For this review, take the finished solid that the model builds, in its own axes (mm). A direction names the side the tool comes from. Give positions to 0.01 mm unless a question says otherwise; leave off trailing zeros. Order: outer loops, then holes, each group sorted by start corner. A loop starts at its lowest first (then second) coordinate and runs counter-clockwise, first axis right, second up. Notation, with made-up numbers: (82, 7.5) -> (103, 7.5) arc R26 ccw to (103, 21.5) -> close; hole circle Ø6 at (-17, 39.25). An arc over 180 degrees is marked (long way). Return JSON: item names as keys, results as strings. Group by question number.
1) Add section A-A (z = 0). State how many separate pieces and enclosed holes the cut face has, then the cut area to 3 significant figures.
2) To check wall thickness, follow line 1 along X through (y, z) = (-8.15, 0) (3 decimals); line 2 along Y through (x, z) = (0, 2.35) (1 decimal); line 3 along X through (y, z) = (-8.5, 1.3). State the ranges of each line that lie inside material, in increasing order.
3) Add section B-B (y = -5.75). Give the boundary of the cut face in (x, z) (1 decimal), then the cut area to 3 significant figures.
4) Insertion check: P1, Ø3, axis at y = 4.5, z = 0, coming from the -X side; P2, Ø2, axis at y = -2, z = 0, coming from the +X side (3 decimals); P3, Ø3, axis at x = -5, z = 0.5, coming from the +Y side; P4, Ø1.9, axis at x = 14.29, z = 0, coming from the -Y side. Each pin has a flat end and moves straight along its axis. Give the tip position at first contact, or say it passes through.
5) For faces 1 (the face through (9.525, -2, 0)), 2 (the face through (-9.525, -2, 0)), 3 (the face through (-9.16, -1.72, 2.16)), 4 (the face through (-17.63, -7.11, -1.896)), 5 (the face through (9.16, -1.77, -2.16)), list the 3-axis set-ups (+Z, -Z, +X, -X, +Y, -Y) from which the entire face can be reached by the end or side of a thin tool; tool diameter is ignored.
from build123d import *

# Parameters (mm, degrees)
EXTRUDE1_DEPTH      = 2.54
EXTRUDE1_DEPTH_BACK = 2.54
SKETCH3_R           = 4.9784
SKETCH4_R           = 1.5875
CUT_EXTRUDE1_DEPTH  = 24.321126052
FILLET1_R           = 1.27
FILLET2_R           = 1.27
CHAMFER1_SIZE       = 0.127
FILLET3_R           = 0.254
CHAMFER2_SIZE       = 0.127


with BuildPart() as part:
    # Sketch3 → Extrude1 (new, two sides: drawn at the far end of the back side and taken through both)
    with BuildSketch(Plane.XY.offset(-EXTRUDE1_DEPTH_BACK)):
        with BuildLine():
            Line((9.525, 0), (9.525, -4.7625))
            Line((9.525, -4.7625), (18.25625, -4.7625))
            Line((18.25625, -4.7625), (18.25625, -9.525))
            Line((18.25625, -9.525), (-18.25625, -9.525))
            Line((-18.25625, -9.525), (-18.25625, -4.7625))
            Line((-18.25625, -4.7625), (-9.525, -4.7625))
            Line((-9.525, -4.7625), (-9.525, 0))
            ThreePointArc((-9.525, 0), (0, 9.525), (9.525, 0))
        make_face()
        Circle(SKETCH3_R, mode=Mode.SUBTRACT)
    extrude(amount=EXTRUDE1_DEPTH + EXTRUDE1_DEPTH_BACK)

    # Sketch4 → Cut-Extrude1 (cut, through all)
    with BuildSketch(Plane(origin=(0, -4.7625, 0), x_dir=(1, 0, 0), z_dir=(0, 1, 0))):
        with Locations(Location((-14.2875, 0, 0), (0, 0, 270))):
            Circle(SKETCH4_R)
        with Locations(Location((14.2875, 0, 0), (0, 0, 270))):
            Circle(SKETCH4_R)
        Polygon((-18.25625, 2.54), (-18.25625, 1.27), (-16.98625, 2.54), align=None)
        Polygon((16.98625, 2.54), (18.25625, 2.54), (18.25625, 1.27), align=None)
        Polygon((18.25625, -2.54), (18.25625, -1.27), (16.98625, -2.54), align=None)
        Polygon((-16.98625, -2.54), (-18.25625, -2.54), (-18.25625, -1.27), align=None)
    extrude(amount=-CUT_EXTRUDE1_DEPTH, mode=Mode.SUBTRACT)

    # Fillet1
    fillet1_edges = [part.edges().sort_by_distance(p)[0] for p in [
        (0, 9.525, -2.54),
        (9.525, -2.38125, -2.54),
        (9.525, -2.38125, 2.54),
        (-9.525, -2.38125, -2.54),
        (0, 9.525, 2.54),
        (-9.525, -2.38125, 2.54),
    ]]
    fillet(fillet1_edges, radius=FILLET1_R)

    # Fillet2
    # the kernel refuses this fillet: 1.27 mm, written as the material it adds along each edge
    with BuildSketch(Plane(origin=(-9.525, -4.7625, -1.27), x_dir=(0, 1, 0), z_dir=(0, 0, 1)), Plane(origin=(9.525, -4.7625, 1.27), x_dir=(0, 1, 0), z_dir=(0, 0, -1))) as fillet2_piece_1:
        with BuildLine():
            CenterArc((FILLET2_R, FILLET2_R), FILLET2_R, 180, 90)
            Line((0, FILLET2_R), (0, 0))
            Line((0, 0), (FILLET2_R, 0))
        make_face()
    extrude(amount=2.54)
    with BuildSketch(Plane(origin=(8.255, -4.7625, -1.27), x_dir=(-0.5976672776328268, 0, 0.8017442392976488), z_dir=(0.8017442392976488, 0, 0.5976672776328268))) as fillet2_piece_2_section:
        with BuildLine():
            CenterArc((1.27 + FILLET2_R, -FILLET2_R), FILLET2_R, 90, 90)
            Line((1.27 + FILLET2_R, 0), (1.27, 0))
            Line((1.27, 0), (1.27, -FILLET2_R))
        make_face()
    fillet2_piece_2 = revolve(axis=Axis((8.255, -4.7625, -1.27), (0, -1, 0)), revolution_arc=233.296989237, mode=Mode.PRIVATE)
    fillet2_piece_2 = split(fillet2_piece_2, bisect_by=Plane(origin=(9.207422318, -4.366731678, -2.54), z_dir=(0, 0, 1)), keep=Keep.TOP, mode=Mode.PRIVATE)
    add(fillet2_piece_2)
    with BuildSketch(Plane(origin=(-8.255, -4.7625, -1.27), x_dir=(0.5976672776328281, 0, 0.8017442392976479), z_dir=(-0.8017442392976479, 0, 0.5976672776328281))) as fillet2_piece_3_section:
        with BuildLine():
            CenterArc((1.27 + FILLET2_R, FILLET2_R), FILLET2_R, 180, 90)
            Line((1.27, FILLET2_R), (1.27, 0))
            Line((1.27, 0), (1.27 + FILLET2_R, 0))
        make_face()
    fillet2_piece_3 = revolve(axis=Axis((-8.255, -4.7625, -1.27), (0, 1, 0)), revolution_arc=233.296989237, mode=Mode.PRIVATE)
    fillet2_piece_3 = split(fillet2_piece_3, bisect_by=Plane(origin=(-9.207422451, -4.366732131, -2.54), z_dir=(0, 0, 1)), keep=Keep.TOP, mode=Mode.PRIVATE)
    add(fillet2_piece_3)
    with BuildSketch(Plane(origin=(8.255, -4.7625, 1.27), x_dir=(1, 0, 0), z_dir=(0, 0, -1))) as fillet2_piece_4_section:
        with BuildLine():
            CenterArc((1.27 + FILLET2_R, -FILLET2_R), FILLET2_R, 90, 90)
            Line((1.27 + FILLET2_R, 0), (1.27, 0))
            Line((1.27, 0), (1.27, -FILLET2_R))
        make_face()
    fillet2_piece_4 = revolve(axis=Axis((8.255, -4.7625, 1.27), (0, -1, 0)), revolution_arc=233.296989237, mode=Mode.PRIVATE)
    fillet2_piece_4 = split(fillet2_piece_4, bisect_by=Plane(origin=(9.207422382, -4.366731938, 2.54), z_dir=(0, 0, -1)), keep=Keep.TOP, mode=Mode.PRIVATE)
    add(fillet2_piece_4)
    with BuildSketch(Plane(origin=(-8.255, -4.7625, 1.27), x_dir=(-1, 0, 0), z_dir=(0, 0, -1))) as fillet2_piece_5_section:
        with BuildLine():
            CenterArc((1.27 + FILLET2_R, FILLET2_R), FILLET2_R, 180, 90)
            Line((1.27, FILLET2_R), (1.27, 0))
            Line((1.27, 0), (1.27 + FILLET2_R, 0))
        make_face()
    fillet2_piece_5 = revolve(axis=Axis((-8.255, -4.7625, 1.27), (0, 1, 0)), revolution_arc=233.296989237, mode=Mode.PRIVATE)
    fillet2_piece_5 = split(fillet2_piece_5, bisect_by=Plane(origin=(-9.804114567, -4.550028742, 2.54), z_dir=(0, 0, -1)), keep=Keep.TOP, mode=Mode.PRIVATE)
    add(fillet2_piece_5)

    # Chamfer1
    chamfer1_edges = [part.edges().sort_by_distance(p)[0] for p in [
        (-4.9784, 0, 2.54),
        (-4.9784, 0, -2.54),
    ]]
    chamfer(chamfer1_edges, length=CHAMFER1_SIZE)

    # Sketch5 → Revolve1 (revolve)
    with BuildSketch(Plane(origin=(0, 0, 0), x_dir=(0, 0, -1), z_dir=(1, 0, 0))):
        Polygon((-2.286, 4.9784), (-2.286, 4.3561), (-2.54, 4.3561), (-2.54, 3.1115), (-2.286, 3.1115), (-2.286, 2.4892), (2.286, 2.4892), (2.286, 3.1115), (2.54, 3.1115), (2.54, 4.3561), (2.286, 4.3561), (2.286, 4.9784), align=None)
    revolve(axis=Axis((0, 0, 0), (0, 0, 1)))

    # Fillet3
    fillet3_edges = [part.edges().sort_by_distance(p)[0] for p in [
        (0, -2.4892, -2.286),
        (0, -2.4892, 2.286),
    ]]
    fillet(fillet3_edges, radius=FILLET3_R)

    # Chamfer2
    chamfer2_edges = [part.edges().sort_by_distance(p)[0] for p in [
        (0, -4.3561, -2.54),
        (0, -3.1115, -2.54),
        (0, -3.1115, 2.54),
        (0, -4.3561, 2.54),
    ]]
    chamfer(chamfer2_edges, length=CHAMFER2_SIZE)


solid = part.part
Evaluation:
{
 "1": {"separate pieces": "3", "enclosed holes": "1", "area": "358 mm^2"},
 "2": {"line 1": "-18.256 to -15.875, -12.7 to 12.7, 15.875 to 18.256", "line 2": "-9.5 to -5, -4.4 to -3.1, 3.1 to 4.4, 5 to 8.9", "line 3": "-18.23 to -15.2, -13.38 to 13.38, 15.2 to 18.23"},
 "3": {"outline": "(-18.3, -1.3) -> (-17, -2.5) -> (17, -2.5) -> (18.3, -1.3) -> (18.3, 1.3) -> (17, 2.5) -> (-17, 2.5) -> (-18.3, 1.3) -> close; hole circle Ø3.2 at (-14.3, 0); hole circle Ø3.2 at (14.3, 0)", "area": "166 mm^2"},
 "4": {"P1": "x = -9.04", "P2": "x = 9.525", "P3": "y = 8.86", "P4": "through"},
 "5": {"face 1": "+Z, -Z, +X, +Y", "face 2": "+Z, -Z, -X, +Y", "face 3": "+Z, -X, +Y", "face 4": "-Z, -X, +Y, -Y", "face 5": "-Z, +X, +Y"}
}
